Verification items for this drawing (mm, ordinates from the low corner). A direction names the side the tool comes from. Coordinates: 2 decimals unless noted, no trailing zeros. Write each loop counter-clockwise with the first axis right and the second up, starting at its lowest first coordinate (ties: lowest second). Pieces come first, ordered by that corner, then holes. Notation, with made-up numbers: M 30.25,4 L 89.25,4 A12 ccw 89.25,13 Z; hole C -11,-10 d11. An arc over 180 degrees is marked long. Write each question's results on one line, items separated by ' | '.
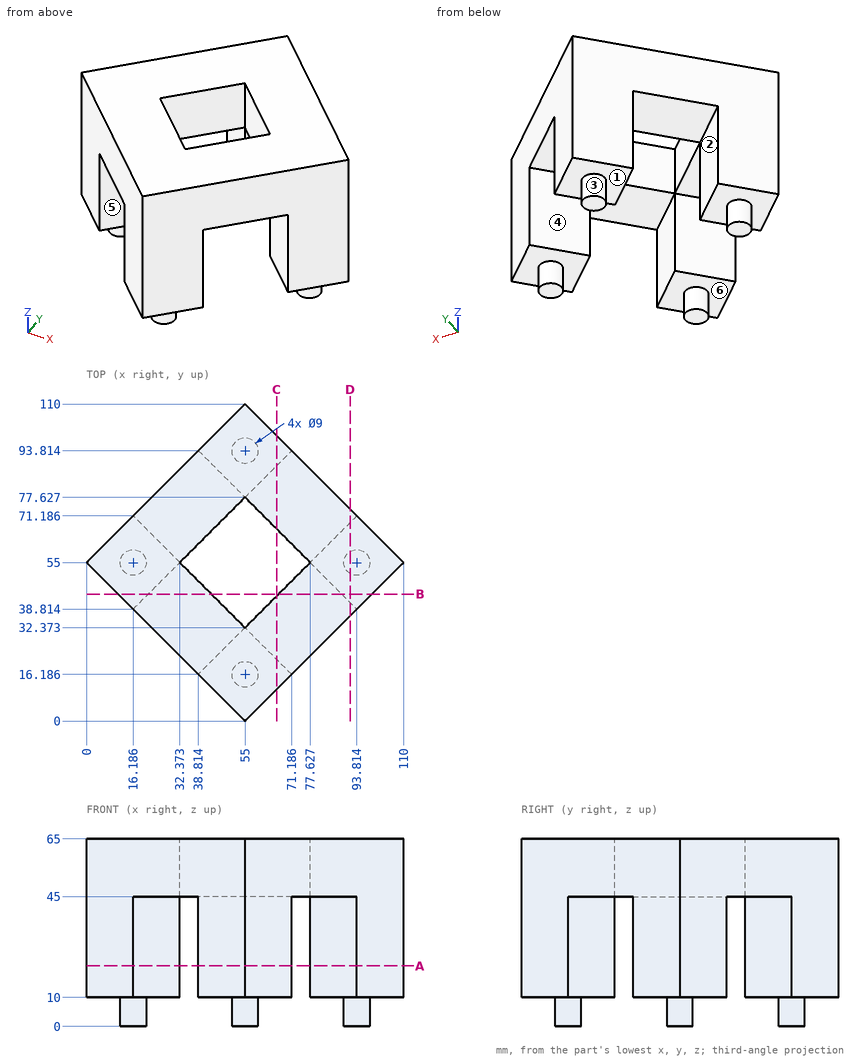
Q1. Sectioned sample at A-A on z = 21. Record the cut outline in (x, y), and give its area (3 significant figures).
Geometry check:
outline: M 0,55 L 16.19,38.81 L 32.37,55 L 16.19,71.19 Z; M 38.81,16.19 L 55,0 L 71.19,16.19 L 55,32.37 Z; M 38.81,93.81 L 55,77.63 L 71.19,93.81 L 55,110 Z; M 77.63,55 L 93.81,38.81 L 110,55 L 93.81,71.19 Z | area: 2,100 mm2
Q2. Mould release check, pull along X, two halves, no side actions. Record for the marked faces 1, 2 and 3: pulls with the +X half, pulls with the -X half, needs draft (parallel to the pull), parting line crosses it, or undercut.
Geometry check:
face 1: needs draft | face 2: undercut | face 3: parting line crosses it
Q3. Sectioned sample at D-D on x = 91.5. Record the cut outline in (y, z), and give its area (3 significant figures).
Geometry check:
outline: M 36.5,45 L 41.13,45 L 41.13,10 L 51.14,10 L 51.14,0 L 58.86,0 L 58.86,10 L 68.87,10 L 68.87,45 L 73.5,45 L 73.5,65 L 36.5,65 Z | area: 1,790 mm2
Q4. Scan lines: probe 1 along Y at (x, z) = (55, 57) (1 decimal); probe 2 along X at (y, z) = (46.5, 52.5) (1 decimal); probe 3 along X at (y, z) = (59, 40) (1 decimal). Record each from-to range of solid material in increasing order.
Geometry check:
probe 1: y = 0 to 32.4, 77.6 to 110 | probe 2: x = 8.5 to 40.9, 69.1 to 101.5 | probe 3: x = 4 to 28.4, 81.6 to 106
Q5. Depth check by flat-ended pin: P1, Ø12, axis at x = 73.5, z = 49.5, coming from the -Y side; P2, Ø19.5, axis at x = 78.5, y = 74.5, coming from the -Z side; P3, Ø3, axis at y = 14, z = 31.5, coming from the -X side. Enter the tip coordinate at first touch or a pass-through.
Geometry check:
P1: stops at y = 12.5 | P2: stops at z = 45 | P3: stops at x = 39.5
Q6. Access from +Z, -Z, +X, -X, +Y, -Y to the whole of each face (thin tool, end or side, straight path). Record for the marked faces 4, 5 and 6.
Geometry check:
face 4: -Z, +Y | face 5: -Z, -Y | face 6: -Z
Q7. Sectioned sample at B-B on y = 44. Record the cut outline in (x, z), and give its area (3 significant figures).
Geometry check:
outline: M 11,10 L 21.37,10 L 21.37,45 L 43.37,45 L 43.37,65 L 11,65 Z; M 66.63,45 L 88.63,45 L 88.63,10 L 99,10 L 99,65 L 66.63,65 Z | area: 2,020 mm2
